Source: three-view drawing plus pictorial views. Frame: mm from the lowest corner of the part. A direction names the side the tool comes from. Coordinates: 2 decimals unless noted, no trailing zeros. Write each loop counter-clockwise with the first axis right and the second up, starting at its lowest first coordinate (ties: lowest second). Pieces come first, ordered by that corner, then holes. Notation, with made-up numbers: (-7, 63) - (10, 63) arc R28 ccw to (10, 100) - close; hole circle Ø2 at (9, -9). An arc over 180 degrees is marked (long way). Put each result on its own line as item: value.
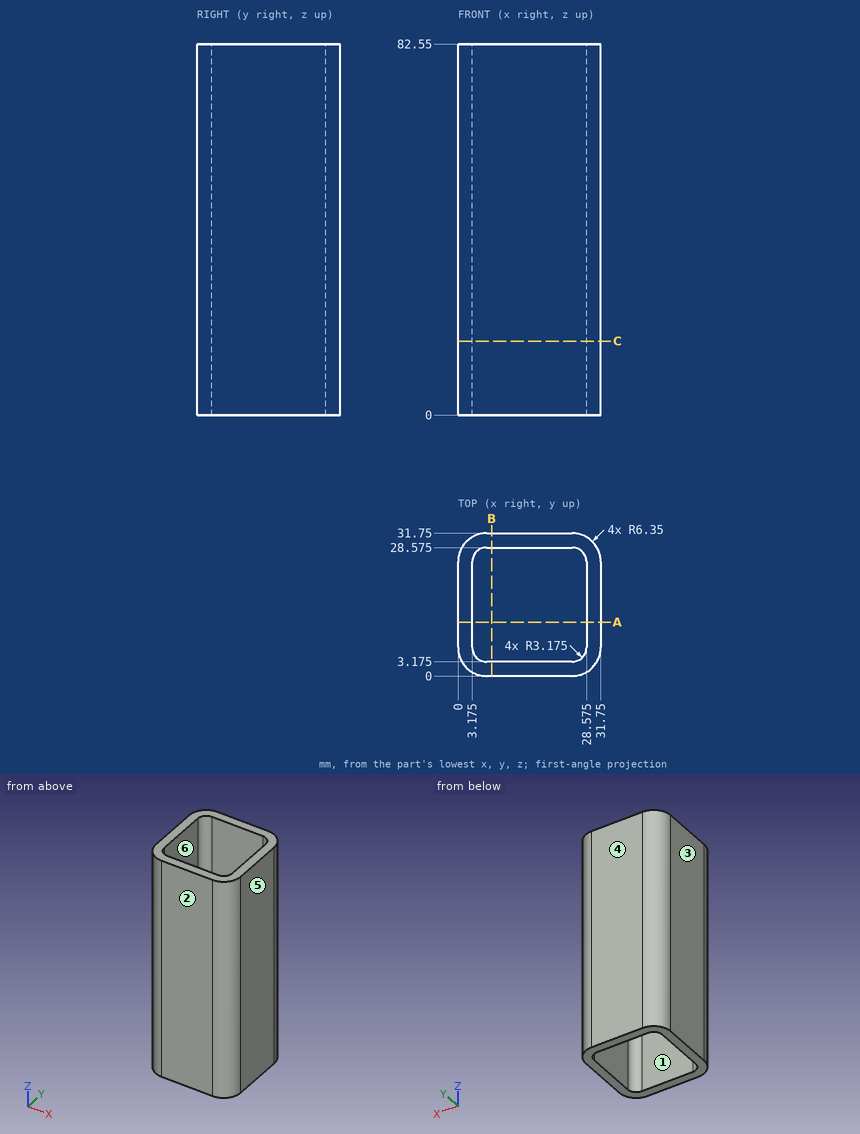
1. Pin query (flat end, axial travel): pin 1 Ø15 at (x, z) = (15.5, 55.5) entering from -Y. Return the tip coordinate at first contact, or that it passes through.
Answer below:
pin 1: stops at y = 0
2. Mould query, pull axis X, two halves, no side actions, for the marked faces 3, 4, 5 and 6. Classes: +X half, -X half, draft (parallel to the pull), parting line (faces both ways), or undercut.
Answer below:
face 3: -X half
face 4: draft
face 5: +X half
face 6: undercut
3. Section query C-C (z = 16.5). Return loops of the section in (x, y) (3 decimals).
Answer below:
outline: (0, 6.35) arc R6.35 ccw to (6.35, 0) - (25.4, 0) arc R6.35 ccw to (31.75, 6.35) - (31.75, 25.4) arc R6.35 ccw to (25.4, 31.75) - (6.35, 31.75) arc R6.35 ccw to (0, 25.4) - close; hole (3.175, 6.35) arc R3.175 ccw to (6.35, 3.175) - (25.4, 3.175) arc R3.175 ccw to (28.575, 6.35) - (28.575, 25.4) arc R3.175 ccw to (25.4, 28.575) - (6.35, 28.575) arc R3.175 ccw to (3.175, 25.4) - close
4. Ray query, probe 1 along X at (y, z) = (18, 37) (3 decimals); probe 2 along X at (y, z) = (26, 12.5). Return the intervals inside material, ascending. Write a range as from..to.
Answer below:
probe 1: x = 0..3.175, 28.575..31.75
probe 2: x = 0.03..3.23, 28.52..31.72
5. Section query A-A (y = 12). Return loops of the section in (x, z) (3 decimals).
Answer below:
outline: (0, 0) - (3.175, 0) - (3.175, 82.55) - (0, 82.55) - close; (28.575, 0) - (31.75, 0) - (31.75, 82.55) - (28.575, 82.55) - close
6. Set-up query: the marked faces 1 and 2. Return all of +Z, -Z, +X, -X, +Y, -Y with unobstructed straight access to the full face (end or side cutting, diameter ignored); none if empty.
Answer below:
face 1: +Z, -Z
face 2: +Z, -Z, +X, -X, -Y
